from build123d import *

# Parameters (mm, degrees)
F1_DEPTH = 177.8
F3_DEPTH = 152.4


with BuildPart() as f1:
    # F0 (on Front) → F1 (new body)
    with BuildSketch(Plane.XZ):
        Polygon((39.275538, 68.027228), (-39.275538, 68.027228), (-78.551077, 0), (-39.275538, -68.027228), (39.275538, -68.027228), (78.551077, 0), align=None)
    extrude(amount=F1_DEPTH)

    # F2 (on face) → F3 (cut)
    with BuildSketch(Plane.XZ.offset(177.8)):
        Polygon((34.086841, 59.04014), (-34.086841, 59.04014), (-68.173682, 0), (-34.086841, -59.04014), (34.086841, -59.04014), (68.173682, 0), align=None)
    extrude(amount=-F3_DEPTH, mode=Mode.SUBTRACT)


solid = f1.part
Verification items for the finished model (mm, model axes). A direction names the side the tool comes from. Round coordinates to 2 decimals unless told otherwise and drop trailing zeros. Loops run counter-clockwise (first coordinate to the right, second up) from the corner with the lowest first, then second, coordinate; pieces in that order, holes last. Notation, with made-up numbers: (73, 58) - (118, 58) arc R19 ccw to (118, 82) - close; hole circle Ø7 at (18.5, 2). An arc over 180 degrees is marked (long way). Use one line per item in the form item = value.
1. Access from +Z, -Z, +X, -X, +Y, -Y to the whole of each face (thin tool, end or side, straight path). Record for faces 1 (the flat face through (-1, -25.4, 1)), 2 (the flat face through (1, -88, 68.027)).
A:
face_1 = -Y
face_2 = +Z, +X, -X, +Y, -Y
2. Section check D-D on z = -48. Record the cut outline in (x, y), and give its area (3 significant figures).
A:
outline = (-50.84, -177.8) - (-40.46, -177.8) - (-40.46, -25.4) - (40.46, -25.4) - (40.46, -177.8) - (50.84, -177.8) - (50.84, 0) - (-50.84, 0) - close
area = 5,750 mm²
3. Section check A-A on x = -14. Record the cut outline in (y, z), and give its area (3 significant figures).
A:
outline = (-177.8, -68.03) - (0, -68.03) - (0, 68.03) - (-177.8, 68.03) - (-177.8, 59.04) - (-25.4, 59.04) - (-25.4, -59.04) - (-177.8, -59.04) - close
area = 6,200 mm²
4. Section check C-C on y = -17. Record the cut outline in (x, z), and give its area (3 significant figures).
A:
outline = (-78.55, 0) - (-39.28, -68.03) - (39.28, -68.03) - (78.55, 0) - (39.28, 68.03) - (-39.28, 68.03) - close
area = 16,000 mm²
5. Scan lines: probe 1 along Z at (x, y) = (2, -95); probe 2 along Y at (x, z) = (12, 6); probe 3 along X at (y, z) = (-44, -30). Record each from-to range of solid material in increasing order.
A:
probe_1 = -68.03 to -59.04, 59.04 to 68.03
probe_2 = -25.4 to 0
probe_3 = -61.23 to -50.85, 50.85 to 61.23
6. Gauge pin test, flat ends, axial feed: pin 1 Ø1 at (x, z) = (-3, 36.5) entering from -Y; pin 2 Ø12 at (y, z) = (-18.5, -26) entering from +X; pin 3 Ø12 at (x, y) = (-49.5, -41) entering from +Z; pin 4 Ø12 at (y, z) = (-67.5, 4.5) entering from -X. Record the tip position at first contact, or that the pin passes through.
A:
pin_1 = -25.4
pin_2 = 67
pin_3 = 60.71
pin_4 = -78.55
7. Draft check along X on faces 3 (the flat face through (-58.64, -87.66, 34.49)), 4 (the flat face through (-1, 0, 1)), 5 (the flat face through (50.892, -102.667, -29.933)). Enter one of: pulls with the +X half, pulls with the -X half, needs draft (parallel to the pull), parting line crosses it, or undercut.
A:
face_3 = pulls with the -X half
face_4 = needs draft
face_5 = undercut
8. Section check B-B on y = -80.5. Record the cut outline in (x, z), and give its area (3 significant figures).
A:
outline = (-78.55, 0) - (-39.28, -68.03) - (39.28, -68.03) - (78.55, 0) - (39.28, 68.03) - (-39.28, 68.03) - close; hole (-68.17, 0) - (-34.09, -59.04) - (34.09, -59.04) - (68.17, 0) - (34.09, 59.04) - (-34.09, 59.04) - close
area = 3,960 mm²
